Can you work these out from the model? Positions are in its coordinate system, mm. A direction names the side the tool comes from. Round coordinates to 2 decimals unless told otherwise and drop trailing zeros. Answer as a JSON object with one key per item and string values.
Autodesk Fusion 360 part; units mm, degrees
sketch "Sketch1" plane through (0, 0, 0) normal (0, 1, 0) x (1, 0, 0)
  line L0 (0, 0) -> (0, -150.6845) construction
  line L1 (0, -150.6845) -> (0, -274) construction
  line L2 (0, 0) -> (910, 0) construction
  line L3 (910, 0) -> (910, -210.245) construction
  arc A0 (0, -274) -> (910, -210.245) centre (1.8405, 6225.9997) ccw
  line L4 (0, -274) -> (0, -244.36)
  line L5 (3, -271.0002) -> (3, -244.36)
  line L6 (910, -210.245) -> (910, -207.2153)
  line L7 (3, -244.36) -> (0, -244.36)
  line L8 (740, -183.31) -> (743, -183.31)
  line L9 (740, -183.31) -> (740, -228.9309)
  line L10 (743, -183.31) -> (743, -228.5871)
  line L11 (740, 0) -> (740, -228.9309) construction
  line L12 (740, -231.9504) -> (740, -347.3942) construction
  arc A1 (743, -228.5871) -> (910, -207.2153) centre (1.8405, 6225.9997) ccw
  line L13 (137, -225.43) -> (140, -225.43)
  line L14 (140, -225.43) -> (140, -269.5311)
  line L15 (137, -225.43) -> (137, -269.5942)
  line L16 (137, 0) -> (137, -269.5942) construction
  line L17 (137, -272.5949) -> (137, -306.2044) construction
  arc A2 (3, -271.0002) -> (137, -269.5942) centre (1.8405, 6225.9997) ccw
  arc A3 (140, -269.5311) -> (740, -228.9309) centre (1.8405, 6225.9997) ccw
  dimension "d1" = 274
  dimension "d2" = 910
  dimension "d3" = 210.245
  dimension "d4" = 6500
  dimension "d5" = 29.64
  dimension "d6" = 170
  dimension "d8" = 3
  dimension "d9" = 183.31
  dimension "d10" = 137
  dimension "d11" = 3
  dimension "d12" = 225.43
revolve "Revolve1" add sketch "Sketch1" angle 360 about axis through (0, 0, 0) along (1, 0, 0)
sketch "Sketch2" plane through (0, 0, 0) normal (-1, 0, 0) x (0, -1, 0)
  circle A0 centre (0, 0) radius 274
  circle A1 centre (0, 0) radius 244.36
  line L0 (0, 0) -> (0, 383.8216) construction
  circle A2 centre (0, 256.86) radius 2
  dimension "d14" = 4
  dimension "d15" = 256.86
extrude "Extrude1" cut sketch "Sketch2" against normal blind 5 contours A2
pattern_circular "C-Pattern1" count 20 over 360 about axis through (1.75, 0, 0) along (1, 0, 0) of "Extrude1"
sketch "Sketch3" plane through (743, 0, 0) normal (1, 0, 0) x (0, 1, 0)
  circle A0 centre (0, 0) radius 183.31
  circle A1 centre (0, 0) radius 228.5871
  line L0 (0, 0) -> (0, 383.9772) construction
  circle A2 centre (0, 200) radius 2
  dimension "d20" = 4
  dimension "d21" = 200
extrude "Extrude2" cut sketch "Sketch3" against normal blind 5 contours A2
pattern_circular "C-Pattern2" count 20 over 360 about axis through (1.75, 0, 0) along (1, 0, 0) of "Extrude2"
equation "d1 = ( 548 / 2 ) * 1 mm"
equation "d3 = ( 420.49 / 2 ) * 1 mm"
Q1. I'm going to push flat-ended pins straight in: pin 1 (4 mm diameter, centred on y = -112.5, z = 168.5, fed in from +X); pin 2 (3 mm diameter, centred on x = 691.5, y = 192, fed in from +Z); pin 3 (2.5 mm diameter, centred on y = 0, z = 200, fed in from -X); pin 4 (10 mm diameter, centred on x = 483, z = -94.5, fed in from -Y) (3 decimals). Where does each tip first touch, or does it pass through?
Determined:
{"pin 1": "x = 743", "pin 2": "z = 141.53", "pin 3": "through", "pin 4": "y = -240.065"}
Q2. We'd pull the mould along X, two halves only. Please class faces 1 (the flat face through (743, -69, -170)), 2 (the flat face through (910, 139, 155)), 3 (the flat face through (140, 218, -61)), 4 (the cylindrical face through (1.479, 165.15, -180.103)): pulls with the +X half, pulls with the -X half, needs draft (parallel to the pull), parting line crosses it, or undercut.
Determined:
{"face 1": "undercut", "face 2": "pulls with the +X half", "face 3": "undercut", "face 4": "needs draft"}
Q3. On a 3-axis mill with a long thin cutter (end or side, diameter ignored), from which of +Z, -Z, +X, -X, +Y, -Y can I reach the whole of each face in a straight line? I mean faces 5 (the flat face through (137, 218, -61)), 6 (the flat face through (0, -245, -1)), 7 (the cylindrical face through (138.52, -67.71, 215.02)). Say none if no direction works.
Determined:
{"face 5": "none", "face 6": "+Z, -Z, -X, +Y, -Y", "face 7": "-X"}
Q4. If I drill on L1, parallel to Y at x = 768, z = -178; L2, parallel to X at y = 201, z = -33.5; L3, parallel to Y at x = 504.5, z = 144, over which ranges is the centre line in solid material (lowest first)? Write a range as [from, to].
Determined:
{"L1": "[-143.58, -138.71], [138.71, 143.58]", "L2": "[740, 743]", "L3": "[-209.89, -206.23], [206.23, 209.89]"}
